Could you check a few things on this model? Use its own coordinates, in mm. A direction names the side the tool comes from. Give positions to 0.01 mm unless a question says otherwise; leave off trailing zeros. Loops run counter-clockwise (first coordinate to the right, second up) from the corner with the lowest first, then second, coordinate; pieces in that order, holes last. Notation, with made-up numbers: (48, 79.5) - (53, 79.5) arc R10 cw to (53, 88.5) - close; hole circle Ø2 at (-30, 14). An arc over 180 degrees is marked (long way). Write each question's results on one line, items separated by ' | '. Start each with the question number.
(1) On a 3-axis mill with a long thin cutter (end or side, diameter ignored), from which of +Z, -Z, +X, -X, +Y, -Y can I reach the whole of each face in a straight line? I mean faces 5 (the face through (-27.5, -1, 3)), 6 (the face through (-26, -1, -22.5)), 7 (the face through (26, -1, 22.5)), 8 (the face through (-17.5, -1, 0)). Say none if no direction works.
(2) Suppose I cut it at D-D (z = -5.5). Please give me the cut outline in (x, y), and give its area (3 significant figures).
(3) Suppose I cut it at C-C (x = 22.5). Please give me the cut outline in (y, z).
(4) For pin 1 (5 mm diameter, centred on x = -22, z = -5.5, fed in from -Y); pin 2 (0.6 mm diameter, centred on x = 7, y = -0.5, fed in from -Z); pin 3 (2.5 mm diameter, centred on x = 22, z = 5.5, fed in from +Y), each with a flat end and sliding along its axis, tell me the tip position at first contact or that it passes through.
(5) Suppose I cut it at B-B (x = -13.5). Please give me the cut outline in (y, z), and give its area (3 significant figures).
(6) If we mould it in two halves opening along Z, with no side actions, what happens to faces 1 (the face through (-19, 0, 0)), 2 (the face through (0, -1, -15)), 3 (the face through (5, -1, 22.5)), 4 (the face through (16.74, -0.99, 18.83))? For each: released by +Z, released by -Z, zero draft, split by the parting line, or undercut.
(7) Suppose I cut it at A-A (z = 1). Please give me the cut outline in (x, y).
(8) I need wall thicknesses on line 1 (X direction, y = -0.45, z = -18.5); line 2 (Z direction, x = -12, y = -1.4); line 3 (X direction, y = -0.5, z = 8). Which ranges of each line are inside material? Lowest first, please.
from build123d import *

# Parameters (mm, degrees)
F0_R     = 2
F1_DEPTH = 2


# Not quite as in the source:
# - ends of sketch curves that miss each other by under 0.0002 mm in the source are joined
# - a feature names something its author has since deleted; it is built from what else it names


with BuildPart() as f1:
    # F0 (on Front) → F1 (new body)
    with BuildSketch(Plane.XZ):
        with BuildLine():
            Line((21.5601722026, 22.5), (-12.5000000166, 22.5))
            Line((-12.5000000166, 22.5), (-5.0000000414, 15))
            Line((-5.0000000414, 15), (17.5, 15))
            Line((17.5, 15), (17.5, -7.5000001159))
            Line((17.5, -7.5000001159), (27.499999851, -17.5))
            Line((27.499999851, -17.5), (27.5, 22.5))
            Line((27.5, 22.5), (24.4017685746, 22.5))
            ThreePointArc((24.4017685746, 22.5), (22.9809703886, 21.4809703886), (21.5601722026, 22.5))
        make_face()
        with Locations((22, -5.5)):
            Circle(F0_R, mode=Mode.SUBTRACT)
        with Locations((22, 5.5)):
            Circle(F0_R, mode=Mode.SUBTRACT)
        with Locations((18.7383297014, 18.7383297014)):
            Circle(F0_R, mode=Mode.SUBTRACT)
        with BuildLine():
            Line((27.499999851, -17.5), (17.5, -7.5000001159))
            Line((17.5, -7.5000001159), (17.5, -15))
            Line((17.5, -15), (5, -15))
            Line((5, -15), (12.5, -22.5))
            Line((12.5, -22.5), (21.5601722026, -22.5))
            ThreePointArc((21.5601722026, -22.5), (22.9809703886, -21.4809703886), (24.4017685746, -22.5))
            Line((24.4017685746, -22.5), (27.5, -22.5))
            Line((27.5, -22.5), (27.499999851, -17.5))
        make_face()
        with Locations((18.7383297014, -18.7383297014)):
            Circle(F0_R, mode=Mode.SUBTRACT)
        with BuildLine():
            Line((21.5601722026, -22.5), (12.5, -22.5))
            Line((12.5, -22.5), (17.5, -27.5))
            Line((17.5, -27.5), (27.5, -27.5))
            Line((27.5, -27.5), (27.5, -22.5))
            Line((27.5, -22.5), (24.4017685746, -22.5))
            ThreePointArc((24.4017685746, -22.5), (24.461037495, -22.7372464453), (24.4809703886, -22.9809703886))
            ThreePointArc((24.4809703886, -22.9809703886), (22.7372464453, -24.461037495), (21.5601722026, -22.5))
        make_face()
        with BuildLine():
            Line((-17.5, 7.5), (-27.5, 17.5))
            Line((-27.5, 17.5), (-27.5, -22.5))
            Line((-27.5, -22.5), (-24.4017685746, -22.5))
            ThreePointArc((-24.4017685746, -22.5), (-22.9809703886, -21.4809703886), (-21.5601722026, -22.5))
            Line((-21.5601722026, -22.5), (12.5, -22.5))
            Line((12.5, -22.5), (5, -15))
            Line((5, -15), (-17.5, -15))
            Line((-17.5, -15), (-17.5, 7.5))
        make_face()
        with Locations((-18.7383297014, -18.7383297014)):
            Circle(F0_R, mode=Mode.SUBTRACT)
        with Locations((-22, -5.5)):
            Circle(F0_R, mode=Mode.SUBTRACT)
        with Locations((-22, 5.5)):
            Circle(F0_R, mode=Mode.SUBTRACT)
        with BuildLine():
            ThreePointArc((-21.5601722026, 22.5), (-22.9809703886, 21.4809703886), (-24.4017685746, 22.5))
            Line((-24.4017685746, 22.5), (-27.5, 22.5))
            Line((-27.5, 22.5), (-27.5, 17.5))
            Line((-27.5, 17.5), (-17.5, 7.5))
            Line((-17.5, 7.5), (-17.5, 15))
            Line((-17.5, 15), (-5.0000000414, 15))
            Line((-5.0000000414, 15), (-12.5000000166, 22.5))
            Line((-12.5000000166, 22.5), (-21.5601722026, 22.5))
        make_face()
        with Locations((-18.7383297014, 18.7383297014)):
            Circle(F0_R, mode=Mode.SUBTRACT)
        with BuildLine():
            ThreePointArc((-24.4017685746, 22.5), (-23.2246943318, 24.461037495), (-21.4809703886, 22.9809703886))
            ThreePointArc((-21.4809703886, 22.9809703886), (-21.5009032821, 22.7372464453), (-21.5601722026, 22.5))
            Line((-21.5601722026, 22.5), (-12.5000000166, 22.5))
            Line((-12.5000000166, 22.5), (-17.5, 27.5))
            Line((-17.5, 27.5), (-27.5, 27.5))
            Line((-27.5, 27.5), (-27.5, 22.5))
            Line((-27.5, 22.5), (-24.4017685746, 22.5))
        make_face()
    extrude(amount=F1_DEPTH)


solid = f1.part
Output values:
1) face 5: +Z, -Z, -X, +Y, -Y | face 6: -Z, -X, +Y, -Y | face 7: +Z, +X, +Y, -Y | face 8: +Y, -Y
2) outline: (-27.5, -2) - (-24, -2) - (-24, 0) - (-27.5, 0) - close; (-20, -2) - (-17.5, -2) - (-17.5, 0) - (-20, 0) - close; (17.5, -2) - (20, -2) - (20, 0) - (17.5, 0) - close; (24, -2) - (27.5, -2) - (27.5, 0) - (24, 0) - close | area: 24.0 mm2
3) outline: (-2, -27.5) - (0, -27.5) - (0, -24.4) - (-2, -24.4) - close; (-2, -21.56) - (0, -21.56) - (0, -7.44) - (-2, -7.44) - close; (-2, -3.56) - (0, -3.56) - (0, 3.56) - (-2, 3.56) - close; (-2, 7.44) - (0, 7.44) - (0, 21.56) - (-2, 21.56) - close
4) pin 1: y = -2 | pin 2: z = -22.5 | pin 3: through
5) outline: (-2, -22.5) - (0, -22.5) - (0, -15) - (-2, -15) - close; (-2, 15) - (0, 15) - (0, 23.5) - (-2, 23.5) - close | area: 32.0 mm2
6) face 1: zero draft | face 2: undercut | face 3: released by +Z | face 4: undercut
7) outline: (-27.5, -2) - (-17.5, -2) - (-17.5, 0) - (-27.5, 0) - close; (17.5, -2) - (27.5, -2) - (27.5, 0) - (17.5, 0) - close
8) line 1: -27.5 to -20.72, -16.75 to 16.75, 20.72 to 27.5 | line 2: -22.5 to -15, 15 to 22.5 | line 3: -27.5 to -17.5, 17.5 to 27.5
